Could you check a few things on this drawing? It's one solid part, dimensions in mm from its lowest x, y, z. Round coordinates to 2 decimals unless told otherwise and drop trailing zeros. Loops run counter-clockwise (first coordinate to the right, second up) from the corner with the lowest first, then second, coordinate; pieces in that order, holes last. Notation, with made-up numbers: M -9,11 L 43,11 A28 cw 43,41 Z; hole C 11.25,27 d8. An arc over 180 degrees is marked long. Answer as a JSON object with one key per item and string values.
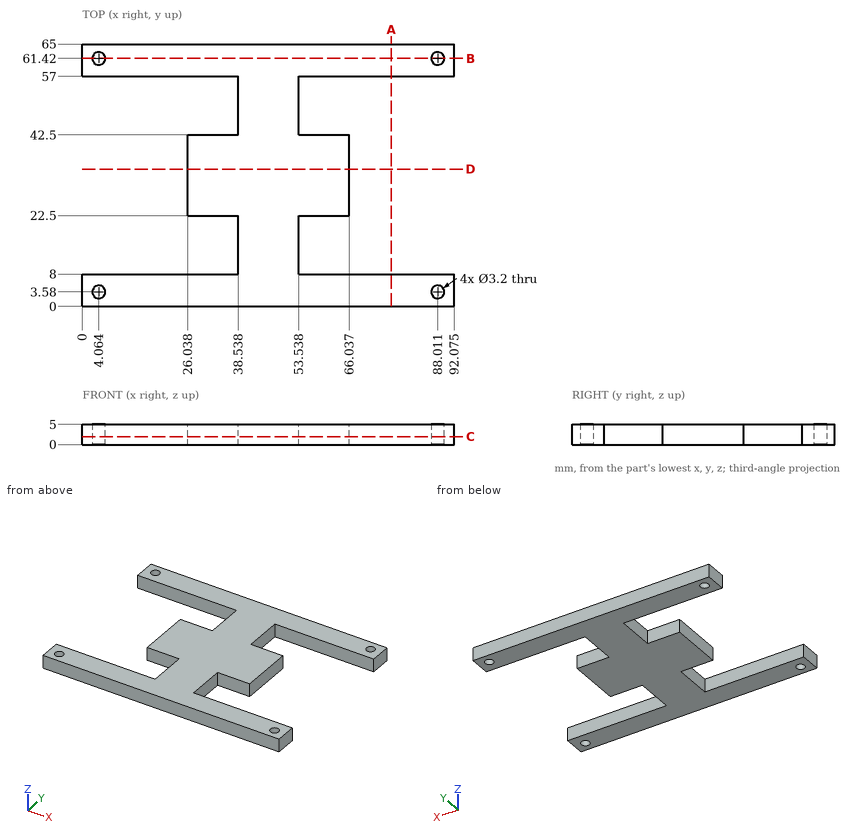
Item 1: I want a section at B-B, the plane y = 61.42. Please give me the cut outline in (x, z) (1 decimal).
Resolved:
{"outline": "M 0,0 L 2.5,0 L 2.5,5 L 0,5 Z; M 5.7,0 L 86.4,0 L 86.4,5 L 5.7,5 Z; M 89.6,0 L 92.1,0 L 92.1,5 L 89.6,5 Z"}
Item 2: I'm going to push flat-ended pins straight in: pin 1 Ø1 at (x, y) = (25.5, 32.5) entering from +Z; pin 2 Ø1.5 at (y, z) = (50, 3) entering from -X; pin 3 Ø2.5 at (y, z) = (36, 2.5) entering from -X; pin 4 Ø1.5 at (y, z) = (53, 3) entering from +X. Where does each tip first touch, or does it pass through?
Resolved:
{"pin 1": "through", "pin 2": "x = 38.54", "pin 3": "x = 26.04", "pin 4": "x = 53.54"}
Item 3: I want a section at A-A, the plane x = 76.5. Please give me the cut outline in (y, z).
Resolved:
{"outline": "M 0,0 L 8,0 L 8,5 L 0,5 Z; M 57,0 L 65,0 L 65,5 L 57,5 Z"}
Item 4: I want a section at C-C, the plane z = 1.95. Please give me the cut outline in (x, y) (1 decimal), then the cut area to 3 significant figures.
Resolved:
{"outline": "M 0,0 L 92.1,0 L 92.1,8 L 53.5,8 L 53.5,22.5 L 66,22.5 L 66,42.5 L 53.5,42.5 L 53.5,57 L 92.1,57 L 92.1,65 L 0,65 L 0,57 L 38.5,57 L 38.5,42.5 L 26,42.5 L 26,22.5 L 38.5,22.5 L 38.5,8 L 0,8 Z; hole C 4.1,3.6 d3.2; hole C 4.1,61.4 d3.2; hole C 88,3.6 d3.2; hole C 88,61.4 d3.2", "area": "2,680 mm²"}
Item 5: I want a section at D-D, the plane y = 34. Please give me the cut outline in (x, z).
Resolved:
{"outline": "M 26.04,0 L 66.04,0 L 66.04,5 L 26.04,5 Z"}
Item 6: Please list where these lines run through material, in increasing order: probe 1 along Y at (x, z) = (33.5, 2.25); probe 2 along Y at (x, z) = (83.5, 2); probe 3 along Y at (x, z) = (4, 2.9). Write a range as from..to.
Resolved:
{"probe 1": "0..8, 22.5..42.5, 57..65", "probe 2": "0..8, 57..65", "probe 3": "0..1.98, 5.18..8, 57..59.82, 63.02..65"}
